Drawing for the job (mm, zero at the part's lowest x, y, z). A direction names the side the tool comes from. Give positions to 0.01 mm unless a question says otherwise; leave off trailing zeros. Loops run counter-clockwise (first coordinate to the right, second up) from the corner with the lowest first, then second, coordinate; pieces in that order, holes last. Notation, with made-up numbers: (-29, 52) -> (3, 52) arc R29 cw to (3, 84) -> close; hole circle Ø5 at (-35, 45.25). An arc over 180 degrees is marked (long way). Write item = value, one per line.
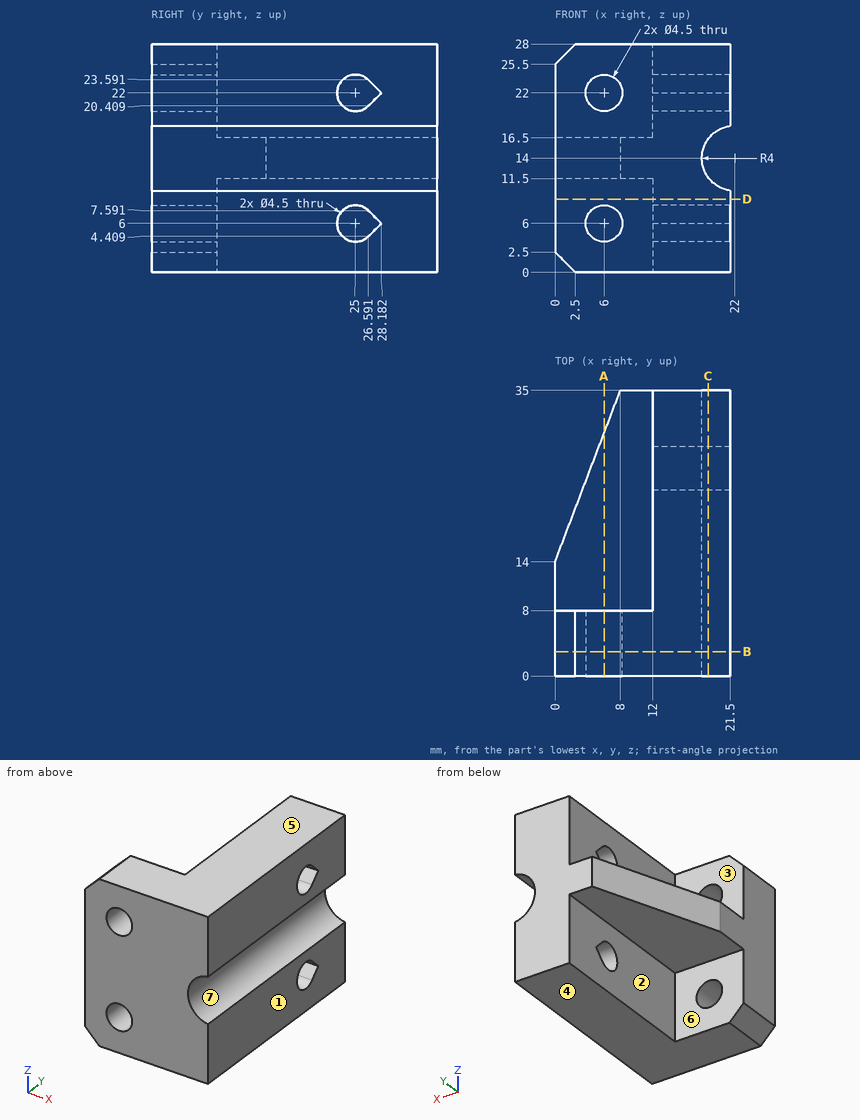
1) Slice it at B-B, the plane y = 3. List the corners of the cut face in (x, z), and give its area (3 significant figures).
Resolved:
outline = (0, 2.5) -> (2.5, 0) -> (21.5, 0) -> (21.5, 10.03) arc R4 cw to (21.5, 17.97) -> (21.5, 28) -> (2.5, 28) -> (0, 25.5) -> close; hole circle Ø4.5 at (6, 6); hole circle Ø4.5 at (6, 22)
area = 543 mm²
2) Which spindle directions (+Z, -Z, +X, -X, +Y, -Y) get a long thin tool onto all of the face, cutting with end or side? Do the marked faces 1, 2 and 3. Say none if no direction does.
Resolved:
face_1 = +Z, -Z, +X, +Y, -Y
face_2 = -Z, -X, +Y
face_3 = +Z, -X, +Y
3) Slice it at C-C, the plane x = 18.75. List the corners of the cut face in (y, z).
Resolved:
outline = (0, 0) -> (35, 0) -> (35, 11.67) -> (0, 11.67) -> close; (0, 16.33) -> (35, 16.33) -> (35, 28) -> (0, 28) -> close; hole (26.59, 4.41) -> (28.18, 6) -> (26.59, 7.59) arc R2.25 ccw (long way) to start; hole (26.59, 20.41) -> (28.18, 22) -> (26.59, 23.59) arc R2.25 ccw (long way) to start
4) Drop flat-ended pins along their axis: P1, Ø3, axis at x = 2.5, y = 22.5, coming from the -Z side; P2, Ø7, axis at x = 6, z = 6, coming from the +Y side; P3, Ø3.5, axis at y = 24.5, z = 24, coming from the -X side. Give the stop position or say it passes through.
Resolved:
P1 = 11.5
P2 = 8
P3 = 12
5) Slice it at A-A, the plane x = 6. List the corners of the cut face in (y, z), and give its area (3 significant figures).
Resolved:
outline = (0, 0) -> (8, 0) -> (8, 3.75) -> (0, 3.75) -> close; (0, 8.25) -> (8, 8.25) -> (8, 11.5) -> (29.75, 11.5) -> (29.75, 16.5) -> (8, 16.5) -> (8, 19.75) -> (0, 19.75) -> close; (0, 24.25) -> (8, 24.25) -> (8, 28) -> (0, 28) -> close
area = 261 mm²
6) Pull direction Z, two halves, no side cores. Call the marked faces 4, 5, 6 and 7: pulls with the +Z half, pulls with the -Z half, needs draft (parallel to the pull), parting line crosses it, or undercut.
Resolved:
face_4 = pulls with the -Z half
face_5 = pulls with the +Z half
face_6 = needs draft
face_7 = undercut
7) Slice it at D-D, the plane z = 9. List the corners of the cut face in (x, y).
Resolved:
outline = (0, 0) -> (21.5, 0) -> (21.5, 35) -> (12, 35) -> (12, 8) -> (0, 8) -> close
8) Drill centre lines: line 1 along Z through (x, y) = (6, 5); line 2 along Y through (x, z) = (2, 17); line 3 along Y through (x, z) = (18.5, 24). Where is each one in solid material? Low to high. Write a range as [from, to].
Resolved:
line_1 = [0, 3.75], [8.25, 19.75], [24.25, 28]
line_2 = [0, 8]
line_3 = [0, 23.97], [26.03, 35]
